The listing builds one solid part. Answer for the finished solid, in the listing's coordinates (mm). A direction names the side the tool comes from. Give positions to 0.01 mm unless a question says otherwise; leave off trailing zeros. Order: outer loops, then holes, each group sorted by start corner. A loop starts at its lowest first (then second) coordinate and runs counter-clockwise, first axis right, second up. Notation, with made-up numbers: (-21.5, 35) - (-17.5, 35) arc R25 cw to (-17.5, 63) - close; hole circle Ø4 at (-36, -28.75). An arc over 180 degrees is marked (long way). Use CSV: the item, a comma, the result in double quotes.
```python
from build123d import *

# Parameters (mm, degrees)
SCHNITT_LINEAR_AUSTRAGEN1_DEPTH = 1.4375


with BuildPart() as part:
    # Skizze1 → Basis-Rotation (revolve)
    with BuildSketch(Plane.XY, mode=Mode.PRIVATE) as basis_rotation_sk:
        with BuildLine():
            Line((0, 12.3), (1.2564, 12.3))
            Line((1.2564, 12.3), (1.5705, 11.9859))
            Line((1.5705, 11.9859), (1.5705, 2.3))
            Line((1.5705, 2.3), (4, 2.3))
            Line((4, 2.3), (4, 2.14295))
            ThreePointArc((4, 2.14295), (2.998207899, 0.849769468), (1.600425673, 0))
            Line((1.600425673, 0), (1.443375673, 0))
            Line((1.443375673, 0), (1.2375, 0.205875673))
            Line((1.2375, 0.205875673), (1.2375, 1.4375))
            Line((1.2375, 1.4375), (0, 2.181065016))
            Line((0, 2.181065016), (0, 12.3))
        make_face()
    revolve(basis_rotation_sk.sketch.rotate(Axis((0, 0, 0), (0, 1, 0)), 90), axis=Axis((0, 0, 0), (0, 1, 0)))  # turned: the seam where the file's is

    # Skizze2 → Schnitt-Linear austragen1 (cut)
    with BuildSketch(Plane(origin=(0, 0, 0), x_dir=(1, 0, 0), z_dir=(0, 1, 0))):
        Polygon((-0.721687836, -1.25), (0.721687836, -1.25), (1.443375673, 0), (0.721687836, 1.25), (-0.721687836, 1.25), (-1.443375673, 0), align=None)
    extrude(amount=SCHNITT_LINEAR_AUSTRAGEN1_DEPTH, mode=Mode.SUBTRACT)


solid = part.part
```
Item 1: The part is cut by section B-B (y = 5.5). Give the vertices of the cut face in (x, z).
Taken from the geometry:
outline,"circle Ø3.14 at (0, 0)"
Item 2: Each of these flat-tipped pins is pushed along its axis until it touches: pin 1 (3 mm diameter, centred on y = 9.5, z = -2, fed in from -X); pin 2 (1 mm diameter, centred on x = -0.5, y = 2, fed in from +Z); pin 3 (1.5 mm diameter, centred on x = -1.5, y = 5, fed in from -Z); pin 4 (4 mm diameter, centred on y = 6, z = -0.5, fed in from +X). Where does it stop, or does it pass through?
Taken from the geometry:
pin 1,"x = -1.49"
pin 2,"z = 4"
pin 3,"z = -1.38"
pin 4,"x = 1.57"
Item 3: Find the intervals of material crossed by line 1 along Y through (x, z) = (-1, 1.25); line 2 along X through (y, z) = (1, -0.5); line 3 along Z through (x, y) = (0.5, 1.75), in increasing order.
Taken from the geometry:
line 1,"0 to 2.3"
line 2,"-3.12 to -1.15, 1.15 to 3.12"
line 3,"-3.74 to -0.51, 0.51 to 3.74"
Item 4: The part is cut by section D-D (x = -3). Give the vertices of the cut face in (y, z), and give its area (3 significant figures).
Taken from the geometry:
outline,"(2.14, -2.65) - (2.3, -2.65) - (2.3, 2.65) - (2.14, 2.65) arc R3.36 ccw to start"
area,"5.60 mm^2"
Item 5: The part is cut by section C-C (z = -2.25). Give the vertices of the cut face in (x, y).
Taken from the geometry:
outline,"(-3.31, 2.14) arc R3.9 ccw to (3.31, 2.14) - (3.31, 2.3) - (-3.31, 2.3) - close"
Item 6: The part is cut by section A-A (y = 1). Give the vertices of the cut face in (x, z), and give its area (3 significant figures).
Taken from the geometry:
outline,"circle Ø6.32 at (0, 0); hole (-1.44, 0) - (-0.72, -1.25) - (0.72, -1.25) - (1.44, 0) - (0.72, 1.25) - (-0.72, 1.25) - close"
area,"25.9 mm^2"
Item 7: The mould has two halves that part along Z. Classify faces 1 (the face through (0, 1, -1.25)), 2 (the face through (-1.06, 7.08, 1.16)), 3 (the face through (0, 2.3, 2)): +Z half, -Z half, draft (parallel to the pull), parting line (faces both ways), or undercut.
Taken from the geometry:
face 1,"undercut"
face 2,"parting line"
face 3,"draft"
Item 8: Which of the six approach directions +Z, -Z, +X, -X, +Y, -Y give full straight-line access (tool end or side, diameter ignored) to faces 4 (the face through (-1.088, 0.709, 0.616)), 5 (the face through (0, 12.3, 0))?
Taken from the geometry:
face 4,"-Y"
face 5,"+Z, -Z, +X, -X, +Y"
